Check sheet for the modelled part. Datum: model origin and axes. Units: mm. Face numbers are marked on the shaded views. A direction names the side the tool comes from. Give positions to 0.01 mm unless a question says otherwise; leave off trailing zeros. Order: outer loops, then holes, each group sorted by start corner. A loop starts at its lowest first (then second) coordinate and runs counter-clockwise, first axis right, second up. Notation, with made-up numbers: (19.25, -10.75) - (76.25, -10.75) arc R18 ccw to (76.25, 10.25) - close; hole circle Ø2 at (-2.5, -7). An arc over 180 degrees is marked (long way). Answer in a Markdown table with one row per item.
from build123d import *

# Parameters (mm, degrees)
BOSS_EXTRUDE1_DEPTH = 100
SKETCH2_W           = 10
SKETCH2_H           = 5
BOSS_EXTRUDE3_DEPTH = 45
SKETCH3_R           = 5
BOSS_EXTRUDE4_DEPTH = 45
SKETCH4_R           = 3.5
CUT_EXTRUDE1_DEPTH  = 45
SKETCH5_W           = 4.6
SKETCH5_H           = 13
BOSS_EXTRUDE5_DEPTH = 25
SKETCH6_R           = 6.1
SKETCH6_R_2         = 2.8
CUT_EXTRUDE2_DEPTH  = 25
SKETCH7_W           = 12.2
SKETCH7_H           = 22.5
CUT_EXTRUDE3_DEPTH  = 3


with BuildPart() as part:
    # Sketch1 → Boss-Extrude1 (new body)
    with BuildSketch(Plane.XY):
        Polygon((-11.5, 5), (11.5, 5), (11.5, 0), (17.5, 0), (17.5, 5), (22.5, 5), (22.5, -10), (-22.5, -10), (-22.5, 5), (-17.5, 5), (-17.5, 0), (-11.5, 0), align=None)
    extrude(amount=BOSS_EXTRUDE1_DEPTH)

    # Sketch2 → Boss-Extrude3 (add)
    with BuildSketch(Plane.ZY.offset(22.5)):
        with Locations((50, -12.5)):
            Rectangle(SKETCH2_W, SKETCH2_H)
    extrude(amount=-BOSS_EXTRUDE3_DEPTH)

    # Sketch3 → Boss-Extrude4 (add)
    with BuildSketch(Plane.ZY.offset(22.5)):
        with Locations((50, -15)):
            Circle(SKETCH3_R)
    extrude(amount=-BOSS_EXTRUDE4_DEPTH)

    # Sketch4 → Cut-Extrude1 (cut)
    with BuildSketch(Plane.ZY.offset(22.5)):
        with Locations((50, -15)):
            Circle(SKETCH4_R)
    extrude(amount=-CUT_EXTRUDE1_DEPTH, mode=Mode.SUBTRACT)

    # Sketch5 → Boss-Extrude5 (add)
    with BuildSketch(Plane(origin=(0, 5, 0), x_dir=(1, 0, 0), z_dir=(0, 1, 0))):
        with Locations((-19.8, -14.5)):
            Rectangle(SKETCH5_W, SKETCH5_H)
        with Locations((19.8, -14.5)):
            Rectangle(SKETCH5_W, SKETCH5_H)
    extrude(amount=BOSS_EXTRUDE5_DEPTH)

    # Sketch6 → Cut-Extrude2 (cut)
    with BuildSketch(Plane(origin=(-17.5, 0, 0), x_dir=(0, 0, -1), z_dir=(1, 0, 0))):
        with Locations((-14.5, 17.8)):
            Circle(SKETCH6_R)
        with Locations((-14.5, 23.9)):
            Circle(SKETCH6_R_2)
    extrude(amount=-CUT_EXTRUDE2_DEPTH, mode=Mode.SUBTRACT)

    # Sketch7 → Cut-Extrude3 (cut)
    with BuildSketch(Plane.ZY.offset(22.1)):
        with Locations((14.5, 22.95)):
            Rectangle(SKETCH7_W, SKETCH7_H)
    extrude(amount=-CUT_EXTRUDE3_DEPTH, mode=Mode.SUBTRACT)


solid = part.part
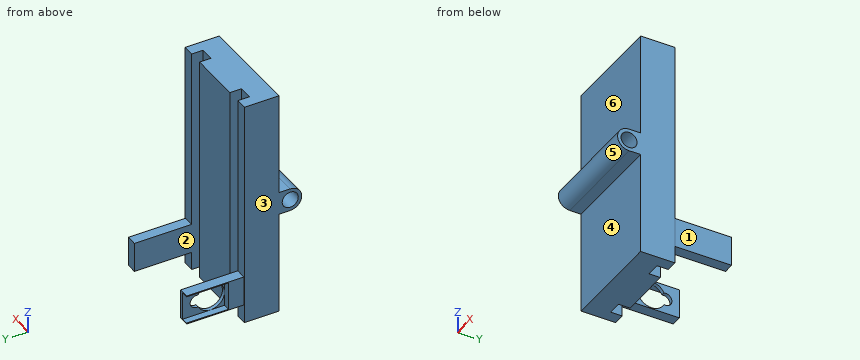
(1) Thickness scan on L1, parallel to Z at x = -18.15, y = 23.9; L2, parallel to Y at x = -18.3, z = 14.5; L3, parallel to Z at x = -18.6, y = 17.8. Record the ranges inside material, lowest first.
Geometry says:
| item | result |
|---|---|
| L1 | 8 to 11.7, 17.3 to 21 |
| L2 | -10 to 11.7, 26.7 to 30 |
| L3 | 8 to 8.4, 20.6 to 21 |
(2) Cross-section at C-C, the plane y = -13. Record the cut outline in (x, z).
Geometry says:
| item | result |
|---|---|
| outline | (-22.5, 45) - (22.5, 45) - (22.5, 47.13) - (-22.5, 47.13) - close; (-22.5, 52.87) - (22.5, 52.87) - (22.5, 55) - (-22.5, 55) - close |
(3) Cross-section at B-B, the plane z = 50. Record the cut outline in (x, y), then the cut area to 3 significant figures.
Geometry says:
| item | result |
|---|---|
| outline | (-22.5, -20) - (22.5, -20) - (22.5, -18.5) - (-22.5, -18.5) - close; (-22.5, -11.5) - (22.5, -11.5) - (22.5, 5) - (17.5, 5) - (17.5, 0) - (11.5, 0) - (11.5, 5) - (-11.5, 5) - (-11.5, 0) - (-17.5, 0) - (-17.5, 5) - (-22.5, 5) - close |
| area | 750 mm² |
(4) Access from +Z, -Z, +X, -X, +Y, -Y to the whole of each face (thin tool, end or side, straight path). Record for the marked faces 4, 5 and 6.
Geometry says:
| item | result |
|---|---|
| face 4 | -Z, +X, -X, -Y |
| face 5 | +X, -X, -Y |
| face 6 | +Z, +X, -X, -Y |
(5) Cross-section at A-A, the plane x = 0.5. Record the cut outline in (y, z).
Geometry says:
| item | result |
|---|---|
| outline | (-15, 45) - (-10, 45) - (-10, 0) - (5, 0) - (5, 100) - (-10, 100) - (-10, 55) - (-15, 55) arc R5 ccw to start; hole circle Ø7 at (-15, 50) |
(6) Mould release check, pull along X, two halves, no side actions. Record for the marked faces 1, 2 and 3: pulls with the +X half, pulls with the -X half, needs draft (parallel to the pull), parting line crosses it, or undercut.
Geometry says:
| item | result |
|---|---|
| face 1 | pulls with the +X half |
| face 2 | undercut |
| face 3 | pulls with the -X half |
(7) Gauge pin test, flat ends, axial feed: P1, Ø5, axis at x = 5.5, z = 44, coming from the -Y side; P2, Ø3.5, axis at x = -20.5, y = 23.5, coming from the +Z side; P3, Ø1.4, axis at x = -20, y = 20.5, coming from the -Z side. Record the tip position at first contact, or that the pin passes through.
Geometry says:
| item | result |
|---|---|
| P1 | y = -18.57 |
| P2 | z = 21 |
| P3 | z = 8 |
